Check sheet for the modelled part. Datum: model origin and axes. Units: mm. Face numbers are marked on the shaded views. A direction names the side the tool comes from. Round coordinates to 2 decimals unless told otherwise and drop trailing zeros. Write each loop counter-clockwise with the first axis right and the second up, starting at its lowest first coordinate (ties: lowest second). Pieces come first, ordered by that corner, then holes. Notation, with made-up numbers: (39, -2) - (95, -2) arc R23 ccw to (95, 24) - close; hole circle Ø11 at (14.25, 62.25). An arc over 180 degrees is marked (long way). Use one line per item in the form item = value. Start each with the question number.
1) Section check A-A (x = -14). Record the boundary of the cut face in (y, z), then the cut area to 3 significant figures.
2) Set-up check for the marked faces 1 and 2: record each of +Z, -Z, +X, -X, +Y, -Y from which the full face is reachable in a straight line by a thin tool's end or side.
3) Section check D-D (y = 15.25). Record the boundary of the cut face in (x, z), then the cut area to 3 significant figures.
4) Scan lines: probe 1 along Y at (x, z) = (-12, 1.75); probe 2 along Z at (x, y) = (10.5, 17). Record each from-to range of solid material in increasing order.
5) Section check B-B (y = 3.5). Record the boundary of the cut face in (x, z).
6) Gauge pin test, flat ends, axial feed: P1, Ø5, axis at x = -0.5, y = 9, coming from the +Z side; P2, Ø1.5, axis at x = -4, z = 12.5, coming from the +Y side; P3, Ø6, axis at y = 14, z = 5, coming from the +X side. Record the tip position at first contact, or that the pin passes through.
7) Section check C-C (x = -2). Record the boundary of the cut face in (y, z).
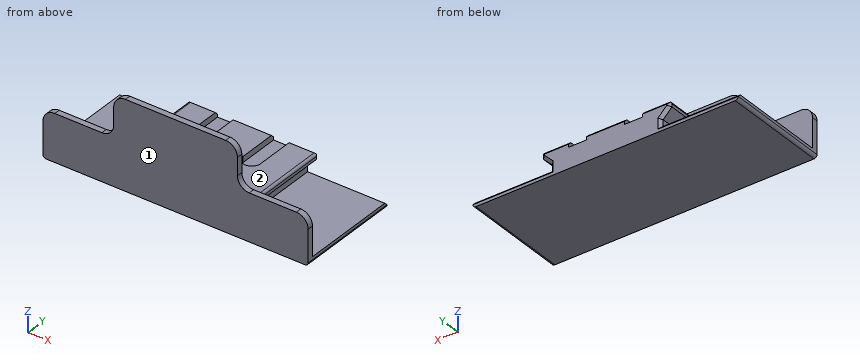
Autodesk Inventor part; units mm, degrees
ref_plane "YZ Plane" through (0, 0, 0) normal (1, 0, 0) x (0, 1, 0)
ref_plane "XZ Plane" through (0, 0, 0) normal (0, 1, 0) x (-1, 0, 0)
ref_plane "XY Plane" through (0, 0, 0) normal (0, 0, 1) x (1, 0, 0)
sketch "Sketch1" plane through (0, 0, 0) normal (0, 0, 1) x (1, 0, 0)
  line L0 (-22.5, 18) -> (22.5, 18)
  line L1 (22.5, 18) -> (22.5, 0)
  line L2 (22.5, 0) -> (-22.5, 0)
  line L3 (-22.5, 0) -> (-22.5, 18)
  point P0 (0, 0)
  point P1 (0, 0)
  dimension "d0" = 18
  dimension "d1" = 45
extrude "Extrusion1" add sketch "Sketch1" along normal blind 1
sketch "Sketch2" plane through (0, 0, 1) normal (0, 0, 1) x (1, 0, 0)
  line L0 (-22.5, 18) -> (-22.5, 0)
  line L1 (-22.5, 0) -> (22.5, 0)
  line L2 (-10.5, 1) -> (10.5, 1)
  line L3 (10.5, 1) -> (10.5, 0)
  line L4 (10.5, 0) -> (-10.5, 0)
  line L5 (-10.5, 0) -> (-10.5, 1)
  point P0 (0, 0)
  point P1 (0, 0)
  dimension "d28" = 21
  dimension "d29" = 1
extrude "Extrusion2" add sketch "Sketch2" along normal blind 14
sketch "Sketch5" plane through (0, 0, 1) normal (0, 0, 1) x (1, 0, 0)
  line L0 (-22.5, 0) -> (22.5, 0)
  line L1 (-22.5, 18) -> (-22.5, 0)
  line L2 (22.5, 0) -> (-22.5, 0)
  line L3 (-22.5, 0) -> (-22.5, 1)
  line L4 (-22.5, 1) -> (22.5, 1)
  line L5 (22.5, 1) -> (22.5, 0)
  line L6 (10.5, 1) -> (-10.5, 1)
extrude "Extrusion5" add sketch "Sketch5" along normal blind 7
sketch "Sketch3" plane through (-22.5, 18, 0) normal (0, 1, 0) x (1, 0, 0)
  line L0 (45, -1) -> (0, -1)
  line L1 (13.1, -1) -> (13.1, -2.1)
  line L2 (13.1, -2.1) -> (11.6, -3.6)
  line L3 (11.6, -3.6) -> (11.6, -4.5)
  line L4 (11.6, -4.5) -> (33.4, -4.5)
  line L5 (33.4, -4.5) -> (33.4, -3.6)
  line L6 (33.4, -3.6) -> (31.9, -2.1)
  line L7 (31.9, -2.1) -> (31.9, -1)
  line L8 (7, -1) -> (43, -1)
  line L9 (22.5, 3) -> (22.5, -18)
  point P0 (22.5, 0)
  dimension "d11" = 135
  dimension "d12" = 1.1
  dimension "d13" = 0.9
  dimension "d14" = 21.8
  dimension "d15" = 3.5
  dimension "d27" = 18.8
extrude "Extrusion3" add sketch "Sketch3" against normal up to surface (18 mm away)
chamfer "Chamfer1" distance 0.5 angle 45 9 edges at (0, 18, 4.5) (10.9, 18, 4.05) (10.15, 18, 2.85) (9.4, 18, 1.55) (15.95, 18, 1) (-10.9, 18, 4.05) (-10.15, 18, 2.85) (-9.4, 18, 1.55) (-15.95, 18, 1)
fillet "Fillet1" radius 0.4 2 edges at (10.9, 9.25, 4.5) (-10.9, 9.25, 4.5)
fillet "Fillet1" radius 0.5 2 edges at (22.5, 9, 0) (-22.5, 9, 0)
sketch "Sketch6" plane through (-10.4, 18, 4) normal (0, 1, 0) x (1, 0, 0)
  line L0 (4.15, -8.7835) -> (7.15, -8.7835)
  line L1 (7.15, -8.7835) -> (7.15, 0.5)
  line L2 (7.15, 0.5) -> (4.15, 0.5)
  line L3 (4.15, 0.5) -> (4.15, -8.7835)
  line L4 (13.65, -8.7835) -> (16.65, -8.7835)
  line L5 (16.65, -8.7835) -> (16.65, 0.5)
  line L6 (16.65, 0.5) -> (13.65, 0.5)
  line L7 (13.65, 0.5) -> (13.65, -8.7835)
  line L8 (5.65, -8.7835) -> (5.65, 0.5) construction
  line L9 (15.15, 0.5) -> (15.15, -8.7835) construction
  line L10 (-0.1, -0.5) -> (20.9, -0.5) construction
  point P0 (10.4, 4)
  dimension "d30" = 3
  dimension "d31" = 1
  dimension "d32" = 9.5
  dimension "d33" = 4.75
extrude "Extrusion6" cut sketch "Sketch6" against normal blind 7
sketch "Sketch7" plane through (-10.5, 1, 4.5) normal (0, 0, 1) x (1, 0, 0)
  line L0 (7.25, 10) -> (4.25, 10)
  arc A0 (4.25, 10) -> (7.25, 10) centre (5.75, 10) ccw
  line L1 (16.75, 10) -> (13.75, 10)
  arc A1 (13.75, 10) -> (16.75, 10) centre (15.25, 10) ccw
  line L2 (7.25, 16.5) -> (7.25, 10)
  line L3 (13.75, 10) -> (13.75, 16.5)
  point P0 (10.5, -1)
extrude "Extrusion7" cut sketch "Sketch7" against normal up to surface (1 mm away)
fillet "Fillet2" radius 2 6 edges at (10.5, 0.5, 8) (22.5, 0.5, 8) (-22.5, 0.5, 8) (-10.5, 0.5, 8) (-10.5, 0.5, 15) (10.5, 0.5, 15)
properties part number "EndSwitchMountingPlate_v02"
Results are:
q1.outline = (0, 0) - (18, 0) - (18, 0.5) - (17.5, 1) - (1, 1) - (1, 8) - (0, 8) - close
q1.area = 24.9 mm²
q2.face_1 = +Z, -Z, +X, -X, -Y
q2.face_2 = +Z, +X, -X, +Y
q3.outline = (-22.5, 0.5) arc R0.5 ccw to (-22, 0) - (22, 0) arc R0.5 ccw to (22.5, 0.5) - (22.5, 1) - (9.4, 1) - (9.4, 2.1) - (10.9, 3.6) - (10.9, 4.1) arc R0.4 ccw to (10.5, 4.5) - (6.25, 4.5) - (6.25, 3.5) - (3.25, 3.5) - (3.25, 4.5) - (-3.25, 4.5) - (-3.25, 3.5) - (-6.25, 3.5) - (-6.25, 4.5) - (-10.5, 4.5) arc R0.4 ccw to (-10.9, 4.1) - (-10.9, 3.6) - (-9.4, 2.1) - (-9.4, 1) - (-22.5, 1) - close
q3.area = 110 mm²
q4.probe_1 = 0 to 1
q4.probe_2 = 0 to 1, 3.2 to 4.5
q5.outline = (-22.5, 0.5) arc R0.5 ccw to (-22, 0) - (22, 0) arc R0.5 ccw to (22.5, 0.5) - (22.5, 1) - (9.4, 1) - (9.4, 2.1) - (10.9, 3.6) - (10.9, 4.1) arc R0.4 ccw to (10.5, 4.5) - (-10.5, 4.5) arc R0.4 ccw to (-10.9, 4.1) - (-10.9, 3.6) - (-9.4, 2.1) - (-9.4, 1) - (-22.5, 1) - close
q6.P1 = 4.5
q6.P2 = 1
q6.P3 = 10.9
q7.outline = (0, 0) - (18, 0) - (18, 4) - (17.5, 4.5) - (1, 4.5) - (1, 15) - (0, 15) - close
